Autodesk Inventor part; units mm, degrees
ref_plane "YZ Plane" through (0, 0, 0) normal (1, 0, 0) x (0, 1, 0)
ref_plane "XZ Plane" through (0, 0, 0) normal (0, 1, 0) x (-1, 0, 0)
ref_plane "XY Plane" through (0, 0, 0) normal (0, 0, 1) x (1, 0, 0)
sketch "Sketch1" plane through (0, 0, 0) normal (1, 0, 0) x (0, 1, 0)
  circle A0 centre (0, 0) radius 40
  dimension "d0" = 80
extrude "Extrusion1" add sketch "Sketch1" along normal blind 20
sketch "Sketch2" plane through (20, 0, 0) normal (1, 0, 0) x (0, 0, -1)
  circle A0 centre (0, 0) radius 40
  line L0 (-11.3165, -38.3658) -> (-7.7264, -29.0325)
  line L1 (-7.7264, -29.0325) -> (2.2736, -29.0325)
  line L2 (2.2736, -29.0325) -> (2.2736, -39.9353)
  line L3 (16.8851, -36.2615) -> (13.3323, -27.4978)
  line L4 (13.3323, -27.4978) -> (20.9893, -21.0659)
  line L5 (20.9893, -21.0659) -> (29.0495, -27.4978)
  line L6 (-34.0034, -21.0659) -> (-26.3463, -14.6339)
  line L7 (-26.3463, -14.6339) -> (-28.141, -4.7963)
  line L8 (-28.141, -4.7963) -> (-39.7114, -4.7963)
  line L9 (-39.7114, 4.7963) -> (-29.7114, 4.7963)
  line L10 (-29.7114, 4.7963) -> (-26.3463, 14.2131)
  line L11 (-26.3463, 14.2131) -> (-33.9262, 21.1899)
  line L12 (35.4673, -18.4951) -> (26.0505, -15.1301)
  line L13 (26.0505, -15.1301) -> (26.0505, -5.1301)
  line L14 (26.0505, -5.1301) -> (39.6697, -5.1301)
  line L15 (-26.3463, 30.0977) -> (-17.7279, 25.026)
  line L16 (-17.7279, 25.026) -> (-8.0547, 27.5618)
  line L17 (-8.0547, 27.5618) -> (-10.9173, 38.4813)
  line L18 (2.2736, 39.9353) -> (2.2736, 30.2694)
  line L19 (2.2736, 30.2694) -> (10.2947, 24.2977)
  line L20 (10.2947, 24.2977) -> (19.1787, 35.1024)
  line L21 (27.4627, 29.0827) -> (20.2021, 22.2063)
  line L22 (20.2021, 22.2063) -> (20.2021, 12.2063)
  line L23 (20.2021, 12.2063) -> (36.9402, 15.3435)
  line L24 (39.9893, -0.9244) -> (29.9893, -0.9244)
  line L25 (29.9893, -0.9244) -> (30.7589, 9.5047)
  line L26 (30.7589, 9.5047) -> (38.0921, 12.2063)
  dimension "d3" = 10
  dimension "d4" = 10
  dimension "d5" = 10
  dimension "d6" = 10
  dimension "d7" = 10
  dimension "d8" = 10
  dimension "d9" = 10
  dimension "d10" = 10
  dimension "d11" = 10
  dimension "d12" = 10
  dimension "d13" = 10
  dimension "d14" = 10
  dimension "d15" = 10
  dimension "d16" = 10
  dimension "d17" = 10
extrude "Extrusion2" cut sketch "Sketch2" against normal blind 20 contours A0 L24 L25 L26 | L23 L22 L21 A0 | A0 L12 L13 L14 | L20 L19 L18 A0 | A0 L3 L4 L5 | L17 L16 L15 A0 | A0 L0 L1 L2 | L11 L10 L9 A0 | A0 L8 L7 L6
sketch "Sketch3" plane through (20, 0, 0) normal (1, 0, 0) x (0, 0, -1)
  arc A0 (-34.0034, -21.0659) -> (-11.3165, -38.3658) centre (0, 0) ccw
  line L0 (-30.137, -26.3014) -> (-22.2204, -21.0659)
  line L1 (-22.2204, -21.0659) -> (-15.2765, -26.3014)
  line L2 (-15.2765, -26.3014) -> (-21.078, -33.9959)
extrude "Extrusion3" cut sketch "Sketch3" against normal blind 20
sketch "Sketch4" plane through (20, 0, 0) normal (1, 0, 0) x (0, 0, -1)
  circle A0 centre (0, 0) radius 5
  dimension "d22" = 10
extrude "Extrusion4" cut sketch "Sketch4" against normal blind 20
properties part number "pinion"
Source: CAD feature listing. Evaluate the final solid. Frame: model axes, mm. A direction names the side the tool comes from. Coordinates: 2 decimals unless noted, no trailing zeros. Loops run counter-clockwise (first coordinate to the right, second up) from the corner with the lowest first, then second, coordinate; pieces in that order, holes last. Notation, with made-up numbers: (21, -16) -> (62, -16) arc R25 cw to (62, 1) -> close; hole circle Ø5 at (87.25, 34.25). An arc over 180 degrees is marked (long way). Answer in a Markdown table with one row per item. Add a question column.
Q1. Pull-direction query (Y, two-part tool) for faces 6 (the face through (10.14, 13.753, -28.454)), 7 (the face through (10.1, 27.6, 22.1)), 8 (the face through (9.86, -3.002, -39.887)); classes: pulls with the +Y half, pulls with the -Y half, needs draft (parallel to the pull), parting line crosses it, or undercut.
Q2. Section A-A on z = 0. Return the cut outline in (x, y).
Q3. Contact query for flat-ended pins moving along their axis: pin 1 Ø2 at (x, z) = (9, 26.5) entering from +Y; pin 2 Ø1.5 at (x, z) = (8, -0.5) entering from -Y; pin 3 Ø11 at (x, z) = (9.5, -34) entering from +Y; pin 4 Ø6 at (y, z) = (-12.5, 14) entering from -X. Output: stop coordinate, or through.
Q4. Reachability of faces 1 (the face through (10, -10, -26.05)), 2 (the face through (10.14, 29.62, -14.67)), 3 (the face through (10.1, -23.7, 26.2)), 4 (the face through (10.14, -23.647, 18.797)), 5 (the face through (10.14, -30.095, 18.137)) from +Z, -Z, +X, -X, +Y, -Y: full face, straight path, thin tool, end or side. Return the list, or none.
Q5. Ray query, line 1 along Y through (x, z) = (14.5, -33) (3 decimals); line 2 along Y through (x, z) = (11, 0); line 3 along Z through (x, y) = (9.25, -22). Return the intervals inside material, ascending.
Q6. Section C-C on z = -34.5. Return the cut outline in (x, y).
Q7. Section B-B on y = 3. Return the cut outline in (x, z), and give its area (3 significant figures).
Q8. Section D-D on y = -6.5. Return the cut outline in (x, z).
Computed values:
| question | item | result |
|---|---|---|
| 1 | face 6 | undercut |
| 1 | face 7 | pulls with the +Y half |
| 1 | face 8 | pulls with the -Y half |
| 2 | outline | (0, -29.03) -> (20, -29.03) -> (20, -5) -> (0, -5) -> close; (0, 5) -> (20, 5) -> (20, 40) -> (0, 40) -> close |
| 3 | pin 1 | stops at y = 30.1 |
| 3 | pin 2 | stops at y = -29.03 |
| 3 | pin 3 | stops at y = 15.34 |
| 3 | pin 4 | stops at x = 0 |
| 4 | face 1 | -Z, +X, -X |
| 4 | face 2 | +X, -X, +Y |
| 4 | face 3 | +X, -X, -Y |
| 4 | face 4 | +X, -X |
| 4 | face 5 | +Z, +X, -X |
| 5 | line 1 | y = -22.605 to -17.613, -5.13 to -0.924, 10.33 to 14.605 |
| 5 | line 2 | y = -29.03 to -5, 5 to 40 |
| 5 | line 3 | z = -33.41 to -22.16, -19.88 to 20.98, 23.63 to 33.41 |
| 6 | outline | (0, -20.24) -> (20, -20.24) -> (20, -18.15) -> (0, -18.15) -> close; (0, -5.13) -> (20, -5.13) -> (20, -0.92) -> (0, -0.92) -> close; (0, 10.88) -> (20, 10.88) -> (20, 14.89) -> (0, 14.89) -> close |
| 7 | outline | (0, -30.28) -> (20, -30.28) -> (20, -4) -> (0, -4) -> close; (0, 4) -> (20, 4) -> (20, 39.89) -> (0, 39.89) -> close |
| 7 | area | 1,240 mm^2 |
| 8 | outline | (0, -26.05) -> (20, -26.05) -> (20, 27.83) -> (0, 27.83) -> close |
